Geometry: final body of the model. Coordinates: model frame, mm. Face numbers are marked on the shaded views. A direction names the side the tool comes from. Round coordinates to 2 decimals unless told otherwise and drop trailing zeros. Write each loop counter-clockwise with the first axis right and the second up, starting at its lowest first coordinate (ties: lowest second). Pieces come first, ordered by that corner, then holes. Notation, with made-up numbers: M 28.25,18 L 83.25,18 A16 cw 83.25,43 Z; hole C 44,-6 d9. An arc over 180 degrees is marked long. Answer as CSV lines item,"result". Start each with the question number.
Q1. Reachability of the marked faces 1 and 2 from +Z, -Z, +X, -X, +Y, -Y: full face, straight path, thin tool, end or side. Return the list, or none.
Q2. Ray query, probe 1 along Y at (x, z) = (-30, 0); probe 2 along X at (y, z) = (74, 0); probe 3 along X at (y, z) = (82, 13). Return the intervals inside material, ascending.
Q3. Section query A-A on z = 0. Output: boundary loops of the cut face in (x, y), and give its area (3 significant figures).
Q4. Section query C-C on y = 40. Output: boundary loops of the cut face in (x, z).
Q5. Section query D-D on z = -15. Output: boundary loops of the cut face in (x, y).
Q6. Section query B-B on x = 0. Output: boundary loops of the cut face in (y, z).
Q7. Mould query, pull axis Y, two halves, no side actions, for the marked faces 3, 4 and 5. Classes: pulls with the +Y half, pulls with the -Y half, needs draft (parallel to the pull), parting line crosses it, or undercut.
Q8. First-contact query: pin 1 (1 mm diameter, centred on x = -10, y = 114.5, fed in from +Z); pin 2 (12 mm diameter, centred on y = 101.5, z = 2.5, fed in from -X); pin 3 (2 mm diameter, centred on x = -0.5, y = 86, fed in from -Z). Flat tips, straight axial feed; report the tip coordinate or a pass-through.
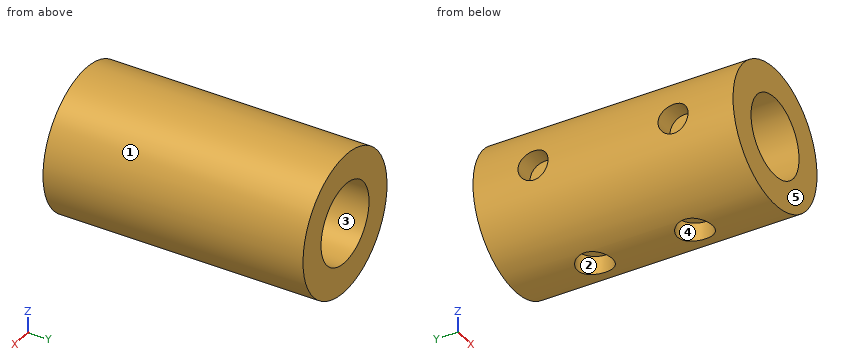
```python
from build123d import *

# Parameters (mm, degrees)
ESQUISSE1_R             = 35
ESQUISSE1_R_2           = 20
BOSS_EXTRU_1_DEPTH      = 130
ENL_V_START             = -25
ESQUISSE2_R             = 8.75
ENL_V_MAT_EXTRU_1_DEPTH = 100
ESQUISSE3_R             = 7.5
ENL_V_MAT_EXTRU_2_DEPTH = 10


with BuildPart() as part:
    # Esquisse1 → Boss.-Extru.1 (new body)
    with BuildSketch(Plane(origin=(0, 0, 0), x_dir=(1, 0, 0), z_dir=(0, 1, 0))):
        with Locations(Location((0, 0, 0), (0, 0, 270))):
            Circle(ESQUISSE1_R)
        with Locations(Location((0, 0, 0), (0, 0, 270))):
            Circle(ESQUISSE1_R_2, mode=Mode.SUBTRACT)
    extrude(amount=BOSS_EXTRU_1_DEPTH)

    # Esquisse2 → Enlèv. mat.-Extru.1 (cut)
    with BuildSketch(Plane.XY.offset(ENL_V_START)):
        with Locations((0, 90)):
            Circle(ESQUISSE2_R)
        with Locations((0, 40)):
            Circle(ESQUISSE2_R)
    extrude(amount=-ENL_V_MAT_EXTRU_1_DEPTH, mode=Mode.SUBTRACT)

    # Esquisse3 → Enlèv. mat.-Extru.2 (cut)
    with BuildSketch(Plane(origin=(-35, 0, 0), x_dir=(0, 0, -1), z_dir=(1, 0, 0))):
        with Locations(Location((0, 100, 0), (0, 0, 180))):
            Circle(ESQUISSE3_R)
        with Locations(Location((0, 30, 0), (0, 0, 180))):
            Circle(ESQUISSE3_R)
    extrude(amount=ENL_V_MAT_EXTRU_2_DEPTH, mode=Mode.SUBTRACT)


solid = part.part
```
Entries:
1,face 1,"+Y, -Y"
1,face 2,"-Z"
2,probe 1,"y = 0 to 22.5, 37.5 to 92.5, 107.5 to 130"
2,probe 2,"x = -35 to -20, 20 to 35"
2,probe 3,"x = -32.5 to -15.2, 15.2 to 32.5"
3,outline,"M -35,0 L -20,0 L -20,130 L -35,130 L -35,107.5 L -25,107.5 L -25,92.5 L -35,92.5 L -35,37.5 L -25,37.5 L -25,22.5 L -35,22.5 Z; M 20,0 L 35,0 L 35,130 L 20,130 Z"
3,area,"3,600 mm^2"
4,outline,"M -8.75,-33.89 L -8.75,-25 L 8.75,-25 L 8.75,-33.89 A35 ccw long Z; hole C 0,0 d40"
5,outline,"M -31.62,0 L -13.23,0 L -13.23,130 L -31.62,130 Z; M 13.23,0 L 31.62,0 L 31.62,130 L 13.23,130 Z"
6,outline,"M 0,-35 L 31.25,-35 L 31.25,-25 L 48.75,-25 L 48.75,-35 L 81.25,-35 L 81.25,-25 L 98.75,-25 L 98.75,-35 L 130,-35 L 130,-20 L 0,-20 Z; M 0,20 L 130,20 L 130,35 L 0,35 Z"
7,face 3,"needs draft"
7,face 4,"undercut"
7,face 5,"pulls with the -Y half"
8,pin 1,"stops at z = 33.69"
8,pin 2,"stops at x = -34.98"
8,pin 3,"stops at z = -25"
